from build123d import *

# Parameters (mm, degrees)
CYLINDER021_R               = 3.7
CYLINDER021_DEPTH           = 8
CYLINDER021_ROLL_ANGLE      = 89.941329
CYLINDER021_PITCH_ANGLE     = 3.606623
CYLINDER021_PLACEMENT_ANGLE = -0.059115
PAD028_DEPTH                = 4
FUSION020_ROLL_ANGLE        = 90
FUSION020_PLACEMENT_ANGLE   = 180
BOX005_W                    = 26
BOX005_H                    = 23
BOX005_DEPTH                = 5
CUT025_ROLL_ANGLE           = -90
CUT025_PLACEMENT_ANGLE      = 180
CYLINDER020_R               = 3.7
CYLINDER020_DEPTH           = 8
CYLINDER020_ROLL_ANGLE      = 89.941329
CYLINDER020_PITCH_ANGLE     = 3.606623
CYLINDER020_PLACEMENT_ANGLE = -0.059115
PAD027_DEPTH                = 4
FUSION019_ROLL_ANGLE        = 90
FUSION019_PLACEMENT_ANGLE   = 180
BOX004_W                    = 26
BOX004_H                    = 19
BOX004_DEPTH                = 5


with BuildPart() as cylinder021:
    # Cylinder021 → Cylinder021 (new body)
    with BuildSketch(Plane.XY):
        Circle(CYLINDER021_R)
    extrude(amount=CYLINDER021_DEPTH)


with BuildPart() as cylinder021_1:
    # Cylinder021 roll: moved
    add(cylinder021.part.rotate(Axis((0, 0, 0), (1, 0, 0)), CYLINDER021_ROLL_ANGLE))


with BuildPart() as cylinder021_2:
    # Cylinder021 pitch: moved
    add(cylinder021_1.part.rotate(Axis((0, 0, 0), (0, 1, 0)), CYLINDER021_PITCH_ANGLE))


with BuildPart() as cylinder021_3:
    # Cylinder021 placement: moved
    add(cylinder021_2.part.moved(Location((21, 34, 6))).rotate(Axis((21, 34, 6), (0, 0, 1)), CYLINDER021_PLACEMENT_ANGLE))


with BuildPart() as obj1:
    # Sketch028 → Pad028 (new body)
    with BuildSketch(Plane.XZ):
        with BuildLine():
            Line((2.271009, 2.906046), (15.224101, 2.179811))
            ThreePointArc((15.224101, -2.179811), (16.5, 0), (15.224101, 2.179811))
            Line((2.224226, -3), (15.224101, -2.179811))
            ThreePointArc((-3.740092, 6.1e-05), (-1.682535, -3.33814), (2.224226, -3))
            Line((-3.709486, 6.1e-05), (-3.740092, 6.1e-05))
            ThreePointArc((2.271009, 2.906046), (-1.628642, 3.324599), (-3.709486, 6.1e-05))
        make_face()
    extrude(amount=PAD028_DEPTH)


with BuildPart() as obj1_1:
    # Body031 placement: moved
    add(obj1.part.moved(Location((21, 34, 6))))

    # Fusion020: union Cylinder021
    add(cylinder021_3.part)


with BuildPart() as obj1_2:
    # Fusion020 roll: moved
    add(obj1_1.part.rotate(Axis((0, 0, 0), (1, 0, 0)), FUSION020_ROLL_ANGLE))


with BuildPart() as obj1_3:
    # Fusion020 placement: moved
    add(obj1_2.part.moved(Location((40, -8, -37))).rotate(Axis((40, -8, -37), (0, 0, 1)), FUSION020_PLACEMENT_ANGLE))


with BuildPart() as cut025:
    # Box005 → Box005 (new body)
    with BuildSketch(Plane(origin=(0, -9, -8), x_dir=(1, 0, 0), z_dir=(0, 0, 1))):
        with Locations((13, 11.5)):
            Rectangle(BOX005_W, BOX005_H)
    extrude(amount=BOX005_DEPTH)

    # Cut025: cut obj1
    add(obj1_3.part, mode=Mode.SUBTRACT)


with BuildPart() as cut025_1:
    # Cut025 roll: moved
    add(cut025.part.rotate(Axis((0, 0, 0), (1, 0, 0)), CUT025_ROLL_ANGLE))


with BuildPart() as cut025_2:
    # Cut025 placement: moved
    add(cut025_1.part.moved(Location((26, 2, 6))).rotate(Axis((26, 2, 6), (0, 0, 1)), CUT025_PLACEMENT_ANGLE))


with BuildPart() as cylinder020:
    # Cylinder020 → Cylinder020 (new body)
    with BuildSketch(Plane.XY):
        Circle(CYLINDER020_R)
    extrude(amount=CYLINDER020_DEPTH)


with BuildPart() as cylinder020_1:
    # Cylinder020 roll: moved
    add(cylinder020.part.rotate(Axis((0, 0, 0), (1, 0, 0)), CYLINDER020_ROLL_ANGLE))


with BuildPart() as cylinder020_2:
    # Cylinder020 pitch: moved
    add(cylinder020_1.part.rotate(Axis((0, 0, 0), (0, 1, 0)), CYLINDER020_PITCH_ANGLE))


with BuildPart() as cylinder020_3:
    # Cylinder020 placement: moved
    add(cylinder020_2.part.moved(Location((21, 34, 6))).rotate(Axis((21, 34, 6), (0, 0, 1)), CYLINDER020_PLACEMENT_ANGLE))


with BuildPart() as obj2:
    # Sketch027 → Pad027 (new body)
    with BuildSketch(Plane.XZ):
        with BuildLine():
            Line((2.271009, 2.906046), (15.224101, 2.179811))
            ThreePointArc((15.224101, -2.179811), (16.5, 0), (15.224101, 2.179811))
            Line((2.224226, -3), (15.224101, -2.179811))
            ThreePointArc((-3.740092, 6.1e-05), (-1.682535, -3.33814), (2.224226, -3))
            Line((-3.709486, 6.1e-05), (-3.740092, 6.1e-05))
            ThreePointArc((2.271009, 2.906046), (-1.628642, 3.324599), (-3.709486, 6.1e-05))
        make_face()
    extrude(amount=PAD027_DEPTH)


with BuildPart() as obj2_1:
    # Body030 placement: moved
    add(obj2.part.moved(Location((21, 34, 6))))

    # Fusion019: union Cylinder020
    add(cylinder020_3.part)


with BuildPart() as obj2_2:
    # Fusion019 roll: moved
    add(obj2_1.part.rotate(Axis((0, 0, 0), (1, 0, 0)), FUSION019_ROLL_ANGLE))


with BuildPart() as obj2_3:
    # Fusion019 placement: moved
    add(obj2_2.part.moved(Location((40, -8, -37))).rotate(Axis((40, -8, -37), (0, 0, 1)), FUSION019_PLACEMENT_ANGLE))


with BuildPart() as fusion021:
    # Box004 → Box004 (new body)
    with BuildSketch(Plane(origin=(0, -9, -8), x_dir=(1, 0, 0), z_dir=(0, 0, 1))):
        with Locations((13, 9.5)):
            Rectangle(BOX004_W, BOX004_H)
    extrude(amount=BOX004_DEPTH)

    # Cut024: cut obj2
    add(obj2_3.part, mode=Mode.SUBTRACT)

    # Fusion021: union Cut025
    add(cut025_2.part)


solid = fusion021.part
Work out the finished part from the listing and answer in its coordinate system (mm). A direction names the side the tool comes from. Give positions to 0.01 mm unless a question says otherwise; leave off trailing zeros. Write each loop counter-clockwise with the first axis right and the second up, starting at its lowest first coordinate (ties: lowest second). Pieces come first, ordered by that corner, then holes. Notation, with made-up numbers: (42, 0) - (55, 0) arc R9 ccw to (55, 4) - close; hole circle Ø6 at (-20.75, -37.5). An arc over 180 degrees is marked (long way). One line per item, written item: value. Start each with the question number.
1. For faces 5 (the flat face through (10.333, 0.547, -4.972)), 6 (the flat face through (13, -5, -3)), 7 (the flat face through (16, 9, 8)), determine the directions among +Z, -Z, +X, -X, +Y, -Y from which every point of the face is accessible in a straight line to the end or side of a thin tool.
2. Consider probe 1 along Y at (x, z) = (17.25, 3.75); probe 2 along Z at (x, y) = (12, 4); probe 3 along Z at (x, y) = (12.75, 0.5). Determine where each line is inside the solid, lowest interval first.
3. Given pin 1 (4 mm diameter, centred on x = 19.5, y = -3.5, fed in from +Z); pin 2 (7.5 mm diameter, centred on x = 15, y = -4, fed in from +Z); pin 3 (5.5 mm diameter, centred on x = 18, z = 8.5, fed in from -Y), each flat-ended and moving along its own axis, determine where each tip first touches the part or whether it passes through.
4. Find section A-A (x = 14). Write down the section's boundary in (y, z).
5. Find section B-B (y = 2.75). Write down the section's boundary in (x, z), then the cut area to 3 significant figures.
6. For a pull along X with two mould halves and no side action, classify faces 1 (the flat face through (13, 1, -8)), 2 (the flat face through (0, 7, -1)), 3 (the flat face through (15.667, 6.972, 5.453)), 4 (the flat face through (10, -2, -7)) as +X half, -X half, draft (parallel to the pull), parting line (faces both ways), or undercut.
7. Find section C-C (z = -2). Write down the section's boundary in (x, y), then the cut area to 3 significant figures.
Geometry results:
1. face 5: +Z
1. face 6: +Z, +X, -X, -Y
1. face 7: -Y
2. probe 1: 5 to 10
2. probe 2: -8 to -3
2. probe 3: -8 to -7
3. pin 1: through
3. pin 2: z = -3
3. pin 3: y = 5
4. outline: (-9, -8) - (10, -8) - (10, 15) - (5, 15) - (5, 10.7) - (9, 10.7) - (9, 5.36) - (5, 5.36) - (5, -3) - (0.75, -3) - (0.75, -7) - (-4.82, -7) - (-4.82, -3) - (-9, -3) - close
5. outline: (0, -8) - (26, -8) - (26, -3) - (0, -3) - close
5. area: 130 mm2
6. face 1: draft
6. face 2: -X half
6. face 3: undercut
6. face 4: undercut
7. outline: (0, 5) - (26, 5) - (26, 10) - (0, 10) - close
7. area: 130 mm2
